```python
from build123d import *

# Parameters (mm, degrees)
F_1_4_0_25_DIAMETER_HOLE6_D     = 6.35
F_1_4_0_25_DIAMETER_HOLE6_DEPTH = 1.902267535
F_1_4_0_25_DIAMETER_HOLE6_TIP   = 1.907732465


with BuildPart() as part:
    # Sketch2 → base_revolve (revolve)
    with BuildSketch(Plane.XY, mode=Mode.PRIVATE) as base_revolve_sk:
        Polygon((20.32, 0), (20.32, -11.43), (0, -11.43), (0, -10.16), (1.27, -10.16), (1.27, -8.89), (0, -8.89), (0, -7.62), (1.27, -7.62), (1.27, -6.35), (0, -6.35), (0, 0), align=None)
    revolve(base_revolve_sk.sketch.rotate(Axis((20.32, 0, 0), (0, -1, 0)), 270), axis=Axis((20.32, 0, 0), (0, -1, 0)))

    # 1/4 (0.25) Diameter Hole6
    with Locations(Plane(origin=(0, 0, 0), x_dir=(1, 0, 0), z_dir=(0, 1, 0))):
        with Locations((8.89, 0)):
            Hole(F_1_4_0_25_DIAMETER_HOLE6_D / 2, depth=F_1_4_0_25_DIAMETER_HOLE6_DEPTH)
            with Locations((0, 0, -(F_1_4_0_25_DIAMETER_HOLE6_DEPTH + F_1_4_0_25_DIAMETER_HOLE6_TIP / 2))):  # 118° drill point
                Cone(0, F_1_4_0_25_DIAMETER_HOLE6_D / 2, F_1_4_0_25_DIAMETER_HOLE6_TIP, mode=Mode.SUBTRACT)


solid = part.part
```
Check sheet for the modelled part. Datum: model origin and axes. Units: mm. A direction names the side the tool comes from. Coordinates: 2 decimals unless noted, no trailing zeros. Write each loop counter-clockwise with the first axis right and the second up, starting at its lowest first coordinate (ties: lowest second). Pieces come first, ordered by that corner, then holes. Notation, with made-up numbers: M 4.25,18 L 60.25,18 A20 cw 60.25,57 Z; hole C -6,32 d7. An arc over 180 degrees is marked long. Write item = value, one per line. Start each with the question number.
1. Sectioned sample at A-A (x = 35.5). Record the cut outline in (y, z).
2. Tool access check on faces 1 (the cylindrical face through (12.06, -0.96, -0.14)), 2 (the cylindrical face through (0.173, -8.246, -2.645)), 3 (the flat face through (2, -8.89, -6)). Record the directions out of +Z, -Z, +X, -X, +Y, -Y that give a thin tool (end or side, any length) a straight path to the whole face; none if there is none.
3. Sectioned sample at B-B (y = -7). Record the cut outline in (x, z).
4. Sectioned sample at C-C (z = -5.5). Record the cut outline in (x, y), then the cut area to 3 significant figures.
5. Mould release check, pull along Z, two halves, no side actions. Record for faces 4 (the flat face through (2, -6.35, -6)), 5 (the conical face through (8.48, -3.48, -0.37)), 6 (the cylindrical face through (31.91, -9.52, -15.12)): pulls with the +Z half, pulls with the -Z half, needs draft (parallel to the pull), parting line crosses it, or undercut.
6. Thickness scan on probe 1 along Y at (x, z) = (15, -19); probe 2 along Z at (x, y) = (8.89, -1) (3 decimals); probe 3 along X at (y, z) = (-1, 14.5). Record the ranges inside material, lowest first.
7. Go/stop test with flat-tipped pins: pin 1 (5 mm diameter, centred on x = 10, y = -1.5, fed in from +Z) (3 decimals); pin 2 (2 mm diameter, centred on y = -6, z = -5.5, fed in from -X); pin 3 (4 mm diameter, centred on x = 22.5, y = -4, fed in from -Z). Record where each tip stops, or that it passes through.
The answers:
q1.outline = M -11.43,-13.51 L -10.16,-13.51 L -10.16,-11.51 L -8.89,-11.51 L -8.89,-13.51 L -7.62,-13.51 L -7.62,-11.51 L -6.35,-11.51 L -6.35,-13.51 L 0,-13.51 L 0,13.51 L -6.35,13.51 L -6.35,11.51 L -7.62,11.51 L -7.62,13.51 L -8.89,13.51 L -8.89,11.51 L -10.16,11.51 L -10.16,13.51 L -11.43,13.51 Z
q2.face_1 = +Y
q2.face_2 = +Y, -Y
q2.face_3 = none
q3.outline = C 20.32,0 d38.1
q4.outline = M 0.76,-11.43 L 39.88,-11.43 L 39.88,-10.16 L 38.56,-10.16 L 38.56,-8.89 L 39.88,-8.89 L 39.88,-7.62 L 38.56,-7.62 L 38.56,-6.35 L 39.88,-6.35 L 39.88,0 L 0.76,0 L 0.76,-6.35 L 2.08,-6.35 L 2.08,-7.62 L 0.76,-7.62 L 0.76,-8.89 L 2.08,-8.89 L 2.08,-10.16 L 0.76,-10.16 Z
q4.area = 440 mm²
q5.face_4 = needs draft
q5.face_5 = undercut
q5.face_6 = parting line crosses it
q6.probe_1 = -11.43 to -10.16, -8.89 to -7.62, -6.35 to 0
q6.probe_2 = -16.801 to -3.175, 3.175 to 16.801
q6.probe_3 = 6.08 to 34.56
q7.pin_1 = 18.755
q7.pin_2 = 0.5
q7.pin_3 = -20.32
